Could you check a few things on this model? Use its own coordinates, in mm. Coordinates: 2 decimals unless noted, no trailing zeros. Write each loop counter-clockwise with the first axis right and the second up, starting at its lowest first coordinate (ties: lowest second). Pieces come first, ordered by that corner, then holes.
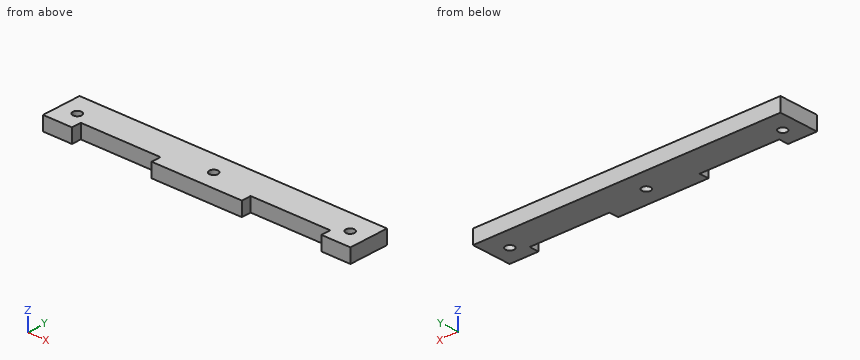
Autodesk Inventor part; units mm, degrees
ref_plane "YZ Plane" through (0, 0, 0) normal (1, 0, 0) x (0, 1, 0)
ref_plane "XZ Plane" through (0, 0, 0) normal (0, 1, 0) x (-1, 0, 0)
ref_plane "XY Plane" through (0, 0, 0) normal (0, 0, 1) x (1, 0, 0)
sketch "Boceto1" plane through (0, 0, 0) normal (0, 0, 1) x (1, 0, 0)
  arc A0 (-67.1173, 21.3488) -> (-68.6673, 19.7988) centre (-67.1173, 19.7988) ccw
  arc A1 (-68.6673, 19.7988) -> (-67.1173, 18.2488) centre (-67.1173, 19.7988) ccw
  arc A2 (-67.1173, 18.2488) -> (-65.5673, 19.7988) centre (-67.1173, 19.7988) ccw
  arc A3 (-65.5673, 19.7988) -> (-67.1173, 21.3488) centre (-67.1173, 19.7988) ccw
  arc A4 (-116.1173, 21.3488) -> (-117.6673, 19.7988) centre (-116.1173, 19.7988) ccw
  arc A5 (-117.6673, 19.7988) -> (-116.1173, 18.2488) centre (-116.1173, 19.7988) ccw
  arc A6 (-116.1173, 18.2488) -> (-114.5673, 19.7988) centre (-116.1173, 19.7988) ccw
  arc A7 (-114.5673, 19.7988) -> (-116.1173, 21.3488) centre (-116.1173, 19.7988) ccw
  arc A8 (-18.1173, 21.3488) -> (-19.6673, 19.7988) centre (-18.1173, 19.7988) ccw
  arc A9 (-19.6673, 19.7988) -> (-18.1173, 18.2488) centre (-18.1173, 19.7988) ccw
  arc A10 (-18.1173, 18.2488) -> (-16.5673, 19.7988) centre (-18.1173, 19.7988) ccw
  arc A11 (-16.5673, 19.7988) -> (-18.1173, 21.3488) centre (-18.1173, 19.7988) ccw
  line L0 (-50.9173, 13.119) -> (-50.9173, 16.5988)
  line L1 (-50.9173, 16.5988) -> (-22.3173, 16.5988)
  line L2 (-22.3173, 16.5988) -> (-22.3173, 13.119)
  line L3 (-22.3173, 13.119) -> (-11.9173, 13.119)
  line L4 (-11.9173, 13.119) -> (-11.9173, 27.4988)
  line L5 (-11.9173, 27.4988) -> (-122.3173, 27.4988)
  line L6 (-122.3173, 27.4988) -> (-122.3173, 13.119)
  line L7 (-122.3173, 13.119) -> (-111.9173, 13.119)
  line L8 (-111.9173, 13.119) -> (-111.9173, 16.5988)
  line L9 (-111.9173, 16.5988) -> (-83.3173, 16.5988)
  line L10 (-83.3173, 16.5988) -> (-83.3173, 13.119)
  line L11 (-83.3173, 13.119) -> (-50.9173, 13.119)
  point P0 (0, 0)
extrude "Extrusión1" add sketch "Boceto1" along normal blind 5
properties part number "carro x lado motor pieza 3"
Item 1: If I drill on line 1 along X through (y, z) = (15.5, 3.3); line 2 along X through (y, z) = (19, 1.7); line 3 along Y through (x, z) = (-103.5, 1.05), over which ranges is the centre line in solid material (lowest first)?
Item 2: I want a section at A-A, the plane z = 2.9. List the corners of the cut face in (x, y) for me.
Item 3: Will this pin go through, and if not, where does the flat tip stop? pin 1 Ø1.5 at (x, z) = (-41, 3) entering from -Y.
Item 4: I want a section at B-B, the plane x = -38.5. List the corners of the cut face in (y, z) for me.
Taken from the geometry:
1. line 1: x = -122.32 to -111.92, -83.32 to -50.92, -22.32 to -11.92
1. line 2: x = -122.32 to -117.45, -114.79 to -68.45, -65.79 to -19.45, -16.79 to -11.92
1. line 3: y = 16.6 to 27.5
2. outline: (-122.32, 13.12) - (-111.92, 13.12) - (-111.92, 16.6) - (-83.32, 16.6) - (-83.32, 13.12) - (-50.92, 13.12) - (-50.92, 16.6) - (-22.32, 16.6) - (-22.32, 13.12) - (-11.92, 13.12) - (-11.92, 27.5) - (-122.32, 27.5) - close; hole circle Ø3.1 at (-116.12, 19.8); hole circle Ø3.1 at (-67.12, 19.8); hole circle Ø3.1 at (-18.12, 19.8)
3. pin 1: stops at y = 16.6
4. outline: (16.6, 0) - (27.5, 0) - (27.5, 5) - (16.6, 5) - close
